For this review, use the dimensioned drawing (mm, ordinates from the lowest corner) and the shaded views. Round coordinates to 2 decimals unless told otherwise and drop trailing zeros. Order: outer loops, then holes, each group sorted by start corner. A loop starts at its lowest first (then second) coordinate and runs counter-clockwise, first axis right, second up. Notation, with made-up numbers: M -12.75,16 L 31.25,16 A36 ccw 31.25,54 Z; hole C 47,-19.75 d4. An arc over 180 degrees is marked long. Answer as CSV lines item,"result". Start each with the question number.
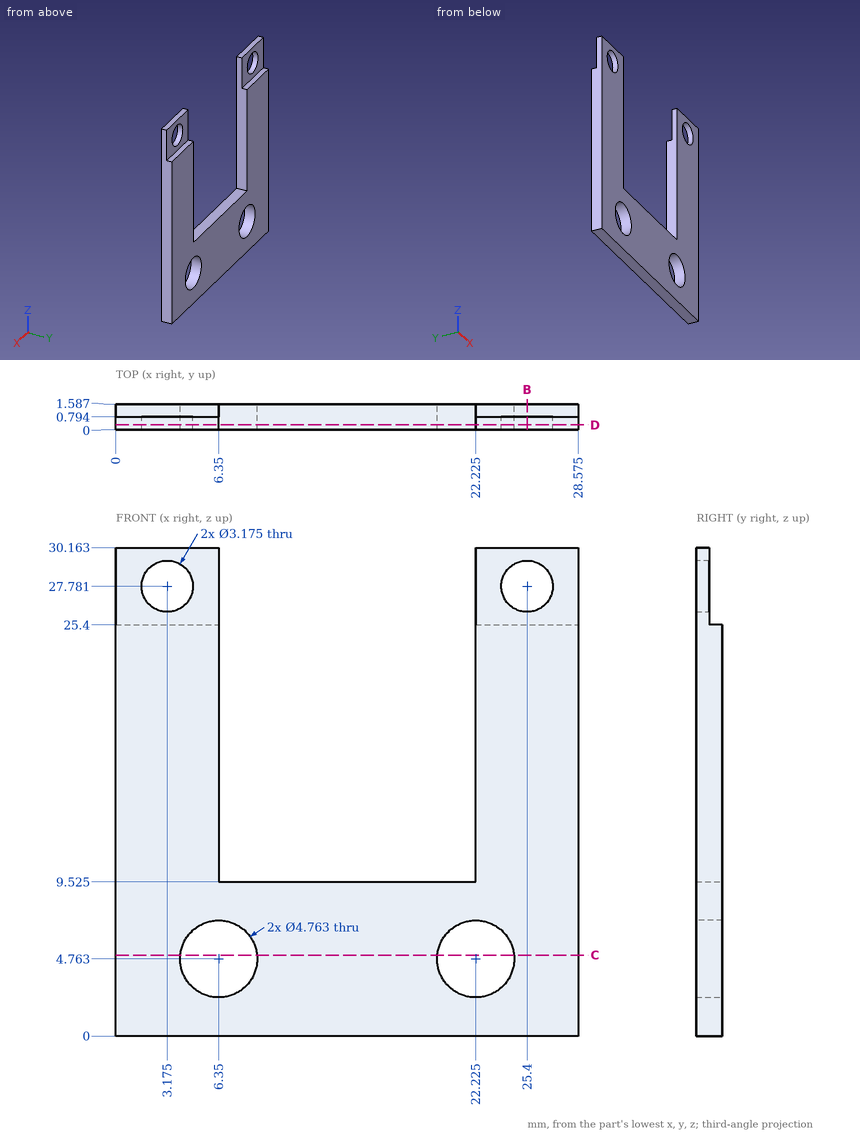
Item 1: Wall thickness on probe 1 along X at (y, z) = (0.2, 5.5) (1 decimal); probe 2 along X at (y, z) = (1.4, 4.5) (1 decimal); probe 3 along Z at (x, y) = (17.75, 0.75) (1 decimal): over which ranges is each line inside the solid? List them lowest first. Write a range as [from, to].
Item 2: Consider section B-B (x = 25.4). State the section outline as (y, z) points.
Item 3: Consider section D-D (y = 0.3). State how many separate pieces and enclosed holes the cut face has, and give its area (3 significant figures).
Item 4: For pin 1 (5 mm diameter, centred on x = 11, z = 17, fed in from +Y); pin 2 (5 mm diameter, centred on x = 3, z = 28.5, fed in from +Y); pin 3 (0.5 mm diameter, centred on x = 17, y = 0.5, fed in from +Z) (1 decimal), all flat-tipped, find the tip position at first contact; note any pin that passes through.
Item 5: Consider section C-C (z = 5). State the section outline as (x, y) points (1 decimal).
Reported:
1,probe 1,"x = [0, 4.1], [8.6, 20], [24.5, 28.6]"
1,probe 2,"x = [0, 4], [8.7, 19.9], [24.6, 28.6]"
1,probe 3,"z = [0, 9.5]"
2,outline,"M 0,0 L 1.59,0 L 1.59,25.4 L 0.79,25.4 L 0.79,26.19 L 0,26.19 Z; M 0,29.37 L 0.79,29.37 L 0.79,30.16 L 0,30.16 Z"
3,separate pieces,"1"
3,enclosed holes,"4"
3,area,"483 mm²"
4,pin 1,"passes through"
4,pin 2,"stops at y = 0.79"
4,pin 3,"stops at z = 9.5"
5,outline,"M 0,0 L 4,0 L 4,1.6 L 0,1.6 Z; M 8.7,0 L 19.9,0 L 19.9,1.6 L 8.7,1.6 Z; M 24.6,0 L 28.6,0 L 28.6,1.6 L 24.6,1.6 Z"
